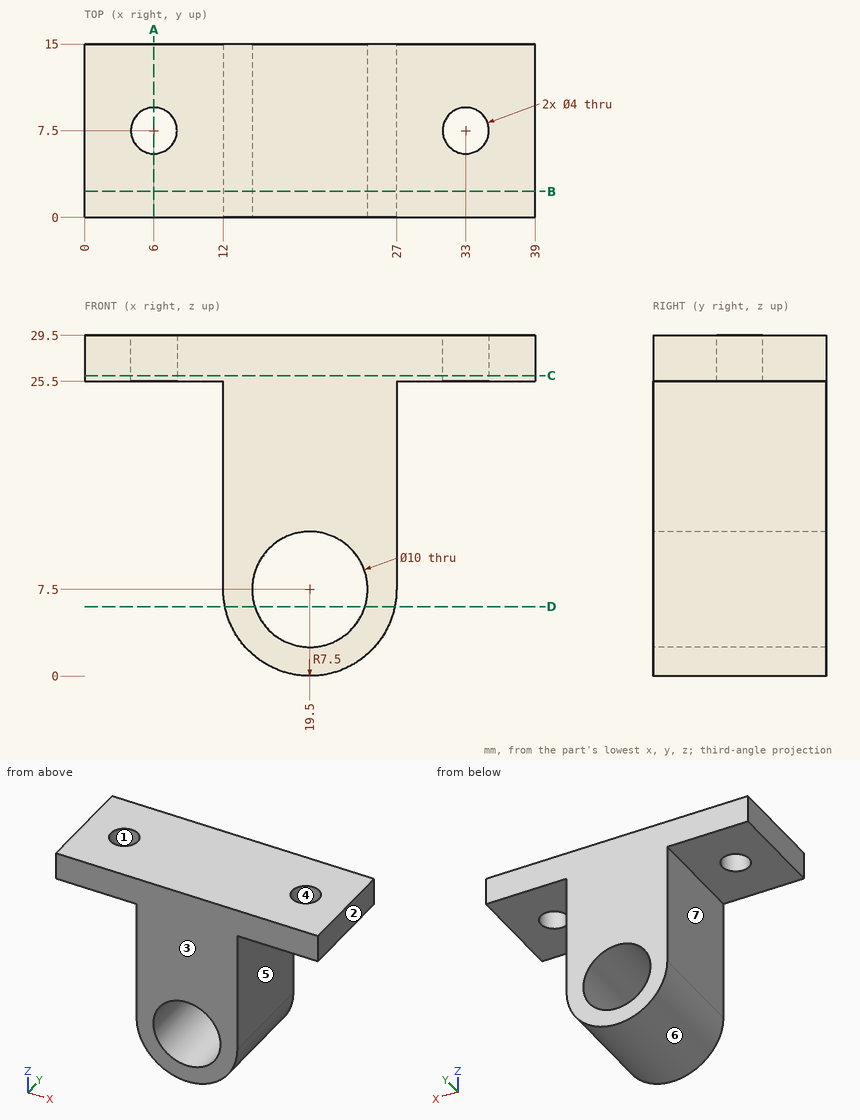
Can you work these out from the drawing? Everything is in mm from the part's minimum corner. A direction names the side the tool comes from. Coordinates: 2 decimals unless noted, no trailing zeros. Loops run counter-clockwise (first coordinate to the right, second up) from the corner with the lowest first, then second, coordinate; pieces in that order, holes last. Notation, with made-up numbers: M 6,-26.5 L 27,-26.5 A23 cw 27,1.5 Z; hole C 68.5,-11.75 d2. An arc over 180 degrees is marked long. One line per item, written item: value.
1. Imagine slicing it at B-B (y = 2.25). List the corners of the cut face in (x, z) for me, and give its area (3 significant figures).
Geometry says:
outline: M 0,25.5 L 12,25.5 L 12,7.5 A7.5 ccw 27,7.5 L 27,25.5 L 39,25.5 L 39,29.5 L 0,29.5 Z; hole C 19.5,7.5 d10
area: 436 mm2
2. On a 3-axis mill with a long thin cutter (end or side, diameter ignored), from which of +Z, -Z, +X, -X, +Y, -Y can I reach the whole of each face in a straight line? I mean the marked faces 5, 6 and 7. Say none if no direction works.
Geometry says:
face 5: -Z, +X, +Y, -Y
face 6: -Z, +Y, -Y
face 7: -Z, -X, +Y, -Y
3. Please list where these lines run through material, in increasing order: probe 1 along Z at (x, y) = (19.5, 8); probe 2 along Y at (x, z) = (6, 27.85); probe 3 along X at (y, z) = (1.75, 24.25).
Geometry says:
probe 1: z = 0 to 2.5, 12.5 to 29.5
probe 2: y = 0 to 5.5, 9.5 to 15
probe 3: x = 12 to 27
4. Imagine slicing it at D-D (z = 6). List the corners of the cut face in (x, y) for me.
Geometry says:
outline: M 12.15,0 L 14.73,0 L 14.73,15 L 12.15,15 Z; M 24.27,0 L 26.85,0 L 26.85,15 L 24.27,15 Z
5. Imagine slicing it at C-C (z = 26). List the corners of the cut face in (x, y) for me.
Geometry says:
outline: M 0,0 L 39,0 L 39,15 L 0,15 Z; hole C 6,7.5 d4; hole C 33,7.5 d4
6. Imagine slicing it at A-A (x = 6). List the corners of the cut face in (y, z) for me, and give its area (3 significant figures).
Geometry says:
outline: M 0,25.5 L 5.5,25.5 L 5.5,29.5 L 0,29.5 Z; M 9.5,25.5 L 15,25.5 L 15,29.5 L 9.5,29.5 Z
area: 44.0 mm2
7. Thinking about a two-plate mould opening in Y: for the marked faces 1, 2, 3 and 4, which applies, +Y half, -Y half, draft (parallel to the pull), parting line (faces both ways), or undercut?
Geometry says:
face 1: undercut
face 2: draft
face 3: -Y half
face 4: undercut
8. Will these pins go through, and if not, where does the flat tip stop? pin 1 Ø1.5 at (x, z) = (6, 23.5) entering from +Y; pin 2 Ø4 at (y, z) = (9.5, 17) entering from +X; pin 3 Ø3.5 at (x, y) = (34.5, 6) entering from -Z; pin 4 Ø4.5 at (y, z) = (4, 16.5) entering from -X.
Geometry says:
pin 1: passes through
pin 2: stops at x = 27
pin 3: stops at z = 25.5
pin 4: stops at x = 12
